For this review, take the finished solid that the model builds, in its own axes (mm). A direction names the side the tool comes from. Give positions to 0.01 mm unless a question says otherwise; leave off trailing zeros. Loops run counter-clockwise (first coordinate to the right, second up) from the corner with the lowest first, then second, coordinate; pieces in that order, holes last. Notation, with made-up numbers: (85, 2) - (112, 2) arc R24 ccw to (112, 12) - close; hole circle Ø9 at (1.25, 78). An arc over 180 degrees is marked (long way). Put each result on its own line as item: value. Start each with the question number.
from build123d import *

# Parameters (mm, degrees)
BOSS_EXTRUDE1_DEPTH = 27.94
SKETCH3_R           = 3.4925
CUT_EXTRUDE1_DEPTH  = 5.08
CIRPATTERN1_COUNT   = 2
CIRPATTERN1_ANGLE   = 30
FILLET2_R           = 6.35
BOSS_EXTRUDE2_DEPTH = 2.54
BOSS_EXTRUDE3_DEPTH = 12.7
FILLET3_R           = 5.08
SKETCH10_R          = 1.905
CUT_EXTRUDE2_DEPTH  = 25.4
CHAMFER2_SIZE       = 2.54
CHAMFER3_SIZE       = 15.24
BOSS_EXTRUDE4_DEPTH = 27.94
CHAMFER4_SIZE       = 12.7
CHAMFER5_SIZE       = 5.08


# Some blends are built 0.0001 mm under size
with BuildPart() as part:
    # Sketch1 → Boss-Extrude1 (new body)
    with BuildSketch(Plane.XY):
        with BuildLine():
            Line((9.358125546, 34.925), (9.861005618, 36.801773982))
            ThreePointArc((9.861005618, 36.801773982), (26.940768363, 26.940768363), (36.801773982, 9.861005618))
            Line((36.801773982, 9.861005618), (34.925, 9.358125546))
            Line((34.925, 9.358125546), (25.566874454, 25.566874454))
            Line((25.566874454, 25.566874454), (9.358125546, 34.925))
        make_face()
    extrude(amount=BOSS_EXTRUDE1_DEPTH)

    # Sketch3 → Cut-Extrude1 (cut)
    with BuildSketch(Plane(origin=(17.4625, 30.245937227, 0), x_dir=(-0.8660254037844386, 0.4999999999999999, 0), z_dir=(-0.49999999999999994, -0.8660254037844387, 0))):
        with Locations(Location((0, -13.97, 0), (0, 0, 180))):
            Circle(SKETCH3_R)
    cut_extrude1 = extrude(amount=-CUT_EXTRUDE1_DEPTH, mode=Mode.SUBTRACT)

    # CirPattern1: Cut-Extrude1 ×2 about axis
    cirpattern1_axis = Axis((0, 0, 27.94), (0, 0, -1))
    for i in range(1, CIRPATTERN1_COUNT):
        add(cut_extrude1.rotate(cirpattern1_axis, i * CIRPATTERN1_ANGLE / (CIRPATTERN1_COUNT - 1)), mode=Mode.SUBTRACT)

    # Fillet2
    fillet2_edges = [part.edges().sort_by_distance(p)[0] for p in [
        (9.609565582, 35.863386991, 0),
        (35.863386991, 9.609565582, 0),
        (25.566874454, 25.566874454, 13.97),
    ]]
    fillet(fillet2_edges, radius=FILLET2_R)

    # Sketch7 → Boss-Extrude2 (add)
    with BuildSketch(Plane.XY.offset(27.94)):
        with BuildLine():
            Line((12.267257994, 3.287001873), (36.801773982, 9.861005618))
            ThreePointArc((36.801773982, 9.861005618), (28.576381723, 25.199214424), (14.387753745, 35.278924901))
            Line((14.387753745, 35.278924901), (4.411323518, 32.605748478))
            Line((4.411323518, 32.605748478), (12.267257994, 3.287001873))
        make_face()
    extrude(amount=BOSS_EXTRUDE2_DEPTH)

    # Sketch8 → Boss-Extrude3 (add)
    with BuildSketch(Plane.XY.offset(30.48)):
        Polygon((4.411323518, 32.605748478), (14.225129913, 35.235349976), (14.882530288, 32.781898378), (5.068723892, 30.152296879), align=None)
        Polygon((7.369625203, 21.565216284), (17.183431598, 24.194817782), (17.840831973, 21.741366183), (8.027025578, 19.111764685), align=None)
    extrude(amount=BOSS_EXTRUDE3_DEPTH)

    # Fillet3
    fillet3_edges = [part.edges().sort_by_distance(p)[0] for p in [
        (14.5538301, 34.008624177, 43.18),
        (17.512131786, 22.968091983, 43.18),
        (7.698325391, 20.338490484, 43.18),
        (4.740023705, 31.379022679, 43.18),
    ]]
    fillet(fillet3_edges, radius=FILLET3_R - 0.0001)  # a hair under: the kernel refuses the full size

    # Sketch10 → Cut-Extrude2 (cut)
    with BuildSketch(Plane(origin=(-4.240232416, 15.824762812, 0), x_dir=(0.9659258262890666, 0.2588190451025272, 0), z_dir=(0.2588190451025272, -0.9659258262890666, 0))):
        with Locations((17.78, 38.1)):
            Circle(SKETCH10_R)
    extrude(amount=-CUT_EXTRUDE2_DEPTH, mode=Mode.SUBTRACT)

    # Chamfer2
    # the kernel refuses this chamfer: 2.54 mm, written as the material it adds along each edge
    with BuildSketch(Plane(origin=(20.697253484, 36.96955026, 27.94), x_dir=(0.00711645652860803, -0.026558977334619874, 0.9996219169112968), z_dir=(-0.9659258262890671, -0.25881904510252557, 0))) as chamfer2_piece_1_section:
        Polygon((CHAMFER2_SIZE * 0.999621916911, CHAMFER2_SIZE * 0.0274958766106), (-CHAMFER2_SIZE * 0.0274958766106, CHAMFER2_SIZE * 0.999621916911), (0, 0), align=None)
    chamfer2_piece_1 = extrude(amount=17.054101493, mode=Mode.PRIVATE)
    chamfer2_piece_1 = chamfer2_piece_1 & Plane(origin=(0, 0, 29.188992539), x_dir=(0.25881904510252113, 0.9659258262890682, 0), z_dir=(0, 0, -1)) * Cylinder(38.1, 45, mode=Mode.PRIVATE)
    chamfer2_piece_1 = split(chamfer2_piece_1, bisect_by=Plane(origin=(9.778458112, 36.493702493, 29.188992539), z_dir=(0.9659258262890693, -0.25881904510251724, 0)), keep=Keep.TOP, mode=Mode.PRIVATE)
    chamfer2_piece_1 = split(chamfer2_piece_1, bisect_by=Plane(origin=(12.882809536, 32.89002275, 29.188992539), z_dir=(0.4999999999999998, 0.8660254037844388, 0)), keep=Keep.TOP, mode=Mode.PRIVATE)
    add(chamfer2_piece_1)

    # Chamfer3
    chamfer3_edges = [part.edges().sort_by_distance(p)[0] for p in [
        (12.267257994, 3.287001873, 29.21),
    ]]
    chamfer(chamfer3_edges, length=CHAMFER3_SIZE)

    # Sketch11 → Boss-Extrude4 (add)
    with BuildSketch(Plane(origin=(0, 0, 27.94), x_dir=(-1, 0, 0), z_dir=(0, 0, -1))):
        with BuildLine():
            Line((-26.41761314, 24.093351826), (-19.258764216, 11.693861766))
            Line((-19.258764216, 11.693861766), (-16.509133559, 13.281361766))
            Line((-16.509133559, 13.281361766), (-24.093351826, 26.41761314))
            ThreePointArc((-24.093351826, 26.41761314), (-25.408479887, 25.408479887), (-26.41761314, 24.093351826))
        make_face()
    extrude(amount=BOSS_EXTRUDE4_DEPTH)

    # Chamfer4
    chamfer4_edges = [part.edges().sort_by_distance(p)[0] for p in [
        (17.883948888, 12.487611766, 0),
    ]]
    chamfer(chamfer4_edges, length=CHAMFER4_SIZE)

    # Chamfer5
    # the kernel refuses this chamfer: 5.08 mm, written as the material it adds along each edge
    with BuildSketch(Plane(origin=(35.40723724, 19.885538351, 27.94), x_dir=(-0.49981095845564816, -0.8656979742248805, 0.027495876610586608), z_dir=(-0.8660254037844388, 0.4999999999999998, 0))) as chamfer5_piece_1_section:
        Polygon((CHAMFER5_SIZE * 0.999621916911, -CHAMFER5_SIZE * 0.0274958766106), (-CHAMFER5_SIZE * 0.0274958766106, -CHAMFER5_SIZE * 0.999621916911), (0, 0), align=None)
    chamfer5_piece_1 = extrude(amount=41.78557159, mode=Mode.PRIVATE)
    chamfer5_piece_1 = split(chamfer5_piece_1, bisect_by=Plane(origin=(8.735724363, 16.466864811, 26.882684671), z_dir=(0.9659258262890666, 0.25881904510252707, 0)), keep=Keep.TOP, mode=Mode.PRIVATE)
    chamfer5_piece_1 = split(chamfer5_piece_1, bisect_by=Plane(origin=(27.739257301, 21.804196991, 26.882684671), z_dir=(-0.8660254037844388, -0.4999999999999997, 0)), keep=Keep.TOP, mode=Mode.PRIVATE)
    chamfer5_piece_1 = split(chamfer5_piece_1, bisect_by=Plane(origin=(22.621869959, 37.485249691, 26.882684671), z_dir=(0.25881904510252557, -0.9659258262890671, 0)), keep=Keep.TOP, mode=Mode.PRIVATE)
    add(chamfer5_piece_1)
    with BuildSketch(Plane(origin=(41.457074789, -1.955759868, 27.94), x_dir=(-0.8656979742248805, -0.49981095845564805, 0.027495876610586608), z_dir=(-0.4999999999999997, 0.8660254037844388, 0))) as chamfer5_piece_2_section:
        Polygon((CHAMFER5_SIZE * 0.999621916911, -CHAMFER5_SIZE * 0.0274958766106), (-CHAMFER5_SIZE * 0.0274958766106, -CHAMFER5_SIZE * 0.999621916911), (0, 0), align=None)
    chamfer5_piece_2 = extrude(amount=43.143072877, mode=Mode.PRIVATE)
    chamfer5_piece_2 = split(chamfer5_piece_2, bisect_by=Plane(origin=(31.353292894, 8.401089511, 26.207782455), z_dir=(-0.2588190451025267, 0.9659258262890668, 0)), keep=Keep.TOP, mode=Mode.PRIVATE)
    chamfer5_piece_2 = split(chamfer5_piece_2, bisect_by=Plane(origin=(32.711409072, 21.441975469, 26.207782455), z_dir=(-0.50000000000019, -0.866025403784329, 0)), keep=Keep.TOP, mode=Mode.PRIVATE)
    add(chamfer5_piece_2)


solid = part.part
1) Mouldability with a two-part tool opening along Y and no side actions: class faces 1 (the cylindrical face through (12.21, 21.53, 36.24)), 2 (the flat face through (24, 12, 27.94)), 3 (the cylindrical face through (9.09, 20.73, 41.65)) as released by +Y, released by -Y, zero draft, split by the parting line, or undercut.
2) Wall thickness on probe 1 along Z at (x, y) = (8.5, 23.75); probe 2 along Z at (x, y) = (18, 33.5); probe 3 along X at (y, z) = (17.5, 23): over which ranges is each line inside the solid? List them lowest first.
3) Machinability: for faces 4 (the flat face through (17.508, 22.985, 34.237)), 5 (the flat face through (14.207, 29.151, 25.436)), 6 (the flat face through (12.208, 22.862, 35.33)), 7 (the flat face through (10.044, 31.486, 35.33)), 8 (the flat face through (13.003, 20.445, 35.33)), which of the approach directions +Z, -Z, +X, -X, +Y, -Y give a long, thin tool a straight path to every point of the face, cutting with its end or side? Answer none if there is none.
4) Take a section at C-C on y = 28. State the section outline as (x, z) points, and give its area (3 significant figures).
5) Take a section at B-B on z = 39. State the section outline as (x, y) points, and give its area (3 significant figures).
6) Insertion check: P1, Ø8.5, axis at x = 22.5, y = 15, coming from the -Z side; P2, Ø6, axis at y = 27, z = 7, coming from the +X side; P3, Ø4, axis at y = 26.5, z = 16, coming from the -X side; P4, Ø12, axis at x = 30.5, y = 33.5, coming from the -Z side. Each pin has a flat end and moves straight along its axis. Give the tip position at first contact, or say it passes through.
7) Take a section at D-D on z = 9.5. State the section outline as (x, y) points (3 decimals).
8) Take a section at A-A on z = 16. State the section outline as (x, y) points (3 decimals), and give its area (3 significant figures).
Answers follow:
1. face 1: undercut
1. face 2: zero draft
1. face 3: released by -Y
2. probe 1: 27.94 to 30.48
2. probe 2: 0 to 10.68, 17.26 to 30.48
2. probe 3: 18.94 to 22.61, 30.06 to 33.84
3. face 4: +Z, +X, +Y
3. face 5: -Z, -X
3. face 6: +Z, -X
3. face 7: +Z, +X
3. face 8: +Z, +X, -Y
4. outline: (5.65, 27.94) - (11.19, 27.94) - (21.35, 22.86) - (21.35, 0) - (25.84, 0) - (25.84, 30.48) - (5.65, 30.48) - close
4. area: 202 mm2
5. outline: (4.49, 32.63) - (5.15, 30.17) - (8.35, 31.03) - (7.7, 33.49) - close; (7.45, 21.59) - (8.1, 19.13) - (11.31, 19.99) - (10.65, 22.45) - close; (10.94, 34.36) - (11.6, 31.9) - (14.8, 32.76) - (14.15, 35.21) - close; (13.9, 23.31) - (14.56, 20.86) - (17.76, 21.72) - (17.11, 24.17) - close
5. area: 33.7 mm2
6. P1: z = 4.13
6. P2: x = 29.59
6. P3: x = 20.49
6. P4: through
7. outline: (9.358, 34.925) - (24.093, 26.418) - (18.109, 16.053) - (20.859, 14.465) - (26.418, 24.093) - (34.925, 9.358) - (36.802, 9.861) arc R38.1 ccw to (9.861, 36.802) - close
8. outline: (9.358, 34.925) - (15.001, 31.667) - (16.536, 34.325) arc R38.1 ccw to (9.861, 36.802) - close; (16.509, 13.281) - (19.259, 11.694) - (26.418, 24.093) - (28.825, 19.924) - (31.483, 21.458) arc R38.1 ccw to (21.458, 31.483) - (19.924, 28.825) - (24.093, 26.418) - close; (31.667, 15.001) - (34.925, 9.358) - (36.802, 9.861) arc R38.1 ccw to (34.325, 16.536) - close
8. area: 118 mm2
